```python
from build123d import *

# Parameters (mm, degrees)
SKETCH1_W           = 30
SKETCH1_H           = 30
BOSS_EXTRUDE1_DEPTH = 30
SKETCH2_R           = 11
CUT_EXTRUDE1_DEPTH  = 15
SKETCH3_R           = 2
BOSS_EXTRUDE2_DEPTH = 10


with BuildPart() as part:
    # Sketch1 → Boss-Extrude1 (new body)
    with BuildSketch(Plane(origin=(0, 0, 0), x_dir=(1, 0, 0), z_dir=(0, 1, 0))):
        Rectangle(SKETCH1_W, SKETCH1_H)
    extrude(amount=BOSS_EXTRUDE1_DEPTH)

    # Sketch2 → Cut-Extrude1 (cut)
    with BuildSketch(Plane(origin=(15, 0, 0), x_dir=(0, 0, -1), z_dir=(1, 0, 0))):
        with Locations((0, 15)):
            Circle(SKETCH2_R)
    extrude(amount=-CUT_EXTRUDE1_DEPTH, mode=Mode.SUBTRACT)

    # Sketch3 → Boss-Extrude2 (add)
    with BuildSketch(Plane(origin=(0, 30, 0), x_dir=(1, 0, 0), z_dir=(0, 1, 0))):
        with Locations(Location((0, 0, 0), (0, 0, 270))):
            Circle(SKETCH3_R)
    extrude(amount=BOSS_EXTRUDE2_DEPTH)


solid = part.part
```
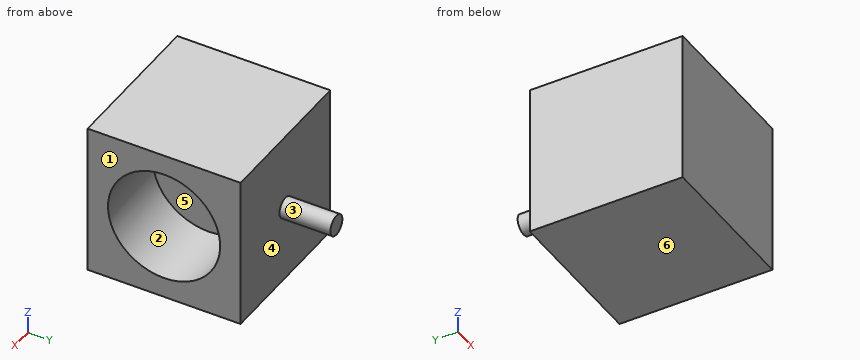
Input: part model. Units: mm. Frame: model coordinates. Face numbers are marked on the shaded views. A direction names the side the tool comes from. Round coordinates to 2 decimals unless told otherwise and drop trailing zeros. Loops run counter-clockwise (first coordinate to the right, second up) from the corner with the lowest first, then second, coordinate; pieces in that order, holes last. Notation, with made-up numbers: (66, 73) -> (94, 73) arc R16 ccw to (94, 78) -> close; hole circle Ø4 at (45.25, -34). An arc over 180 degrees is marked (long way). One line per item, written item: value.
(1) Material intervals for line 1 (Y direction, x = 8.25, z = 0); line 2 (X direction, y = 18, z = 1.5); line 3 (Y direction, x = -3, z = -9), sorted ascending. Write a range as [from, to].
Geometry check:
line 1: [0, 4], [26, 30]
line 2: [-15, 0]
line 3: [0, 30]
(2) Mould query, pull axis Z, two halves, no side actions, for the marked faces 4, 5 and 6. Classes: pulls with the +Z half, pulls with the -Z half, needs draft (parallel to the pull), parting line crosses it, or undercut.
Geometry check:
face 4: needs draft
face 5: undercut
face 6: pulls with the -Z half
(3) Set-up query: the marked faces 1, 2 and 3. Return all of +Z, -Z, +X, -X, +Y, -Y with unobstructed straight access to the full face (end or side cutting, diameter ignored); none if empty.
Geometry check:
face 1: +Z, -Z, +X, +Y, -Y
face 2: +X
face 3: +Y
(4) Section A-A (y = 15). Return the cut outline in (x, z).
Geometry check:
outline: (-15, -15) -> (15, -15) -> (15, -11) -> (0, -11) -> (0, 11) -> (15, 11) -> (15, 15) -> (-15, 15) -> close
(5) Section C-C (x = 4.5). Return the cut outline in (y, z).
Geometry check:
outline: (0, -15) -> (30, -15) -> (30, 15) -> (0, 15) -> close; hole circle Ø22 at (15, 0)
(6) Section D-D (x = -1.25). Return the cut outline in (y, z).
Geometry check:
outline: (0, -15) -> (30, -15) -> (30, -1.56) -> (40, -1.56) -> (40, 1.56) -> (30, 1.56) -> (30, 15) -> (0, 15) -> close
(7) Pin query (flat end, axial travel): pin 1 (1 mm diameter, centred on x = 9, z = 8.5, fed in from +Y); pin 2 (5 mm diameter, centred on y = 11, z = -6.5, fed in from +X). Return the tip coordinate at first contact, or that it passes through.
Geometry check:
pin 1: y = 30
pin 2: x = 0
(8) Section B-B (z = 0). Return the cut outline in (x, y), plus the area to 3 significant figures.
Geometry check:
outline: (-15, 0) -> (15, 0) -> (15, 4) -> (0, 4) -> (0, 26) -> (15, 26) -> (15, 30) -> (2, 30) -> (2, 40) -> (-2, 40) -> (-2, 30) -> (-15, 30) -> close
area: 610 mm2
